Input: part model. Units: mm. Frame: model coordinates. A direction names the side the tool comes from. Coordinates: 2 decimals unless noted, no trailing zeros. Write each loop counter-clockwise with the first axis right and the second up, starting at its lowest first coordinate (ties: lowest second). Pieces come first, ordered by that corner, then holes.
from build123d import *

# Parameters (mm, degrees)
SKETCH1_R           = 3.429
BOSS_EXTRUDE1_DEPTH = 202.2602
BOSS_EXTRUDE2_DEPTH = 6.35
CIRPATTERN1_COUNT   = 2


with BuildPart() as part:
    # Sketch1 → Boss-Extrude1 (new body)
    with BuildSketch(Plane(origin=(0, 0, 0), x_dir=(1, 0, 0), z_dir=(0, 1, 0))):
        with BuildLine():
            Line((19.998392739, 2.54), (-19.998392739, 2.54))
            ThreePointArc((-19.998392739, 2.54), (-31.369, 0), (-19.998392739, -2.54))
            Line((-19.998392739, -2.54), (19.998392739, -2.54))
            ThreePointArc((19.998392739, -2.54), (31.369, 0), (19.998392739, 2.54))
        make_face()
        with Locations(Location((-25.4, 0, 0), (0, 0, 270))):
            Circle(SKETCH1_R, mode=Mode.SUBTRACT)
        with Locations(Location((25.4, 0, 0), (0, 0, 270))):
            Circle(SKETCH1_R, mode=Mode.SUBTRACT)
    extrude(amount=BOSS_EXTRUDE1_DEPTH)

    # Sketch3 → Boss-Extrude2 (add, symmetric)
    with BuildSketch(Plane(origin=(0, 101.1301, 0), x_dir=(1, 0, 0), z_dir=(0, 1, 0))):
        with BuildLine():
            Line((-28.809566389, 4.899369147), (-4.826, 21.59))
            Line((-4.826, 21.59), (4.826, 21.59))
            Line((4.826, 21.59), (28.809566389, 4.899369147))
            ThreePointArc((28.809566389, 4.899369147), (23.85607241, 5.765869284), (19.998392739, 2.54))
            Line((19.998392739, 2.54), (-19.998392739, 2.54))
            ThreePointArc((-19.998392739, 2.54), (-23.85607241, 5.765869284), (-28.809566389, 4.899369147))
        make_face()
    boss_extrude2 = extrude(amount=BOSS_EXTRUDE2_DEPTH, both=True)

    # CirPattern1: Boss-Extrude2 ×2 about axis
    cirpattern1_axis = Axis((0, 0, 0), (0, 1, 0))
    for i in range(1, CIRPATTERN1_COUNT):
        add(boss_extrude2.rotate(cirpattern1_axis, i * 360 / CIRPATTERN1_COUNT))


solid = part.part
Item 1: Pin query (flat end, axial travel): pin 1 Ø8 at (x, y) = (9.5, 24) entering from +Z; pin 2 Ø1 at (x, y) = (-8, 162.5) entering from -Z; pin 3 Ø5.5 at (x, z) = (-14.5, -16.5) entering from +Y. Return the tip coordinate at first contact, or that it passes through.
Item 2: Material intervals for line 1 (X direction, y = 113, z = 0); line 2 (X direction, y = 105.5, z = 0.5); line 3 (X direction, y = 16.5, z = 3), sorted ascending.
Item 3: Access query for faces 1 (the face through (0, 154, 2.54)), 2 (the face through (0, 47, -2.54)), 3 (the face through (0, 107.48, -10)), 4 (the face through (0, 94.78, 10)), 5 (the face through (31.365, 99.714, 0.226)). Directions: +Z, -Z, +X, -X, +Y, -Y. A direction counts if a zero-diameter tool reaches every point of the face in a straight line with its end or side. Return the directions, or none.
Item 4: Section query D-D, the plane x = -1.5. Return loops of the section in (y, z), then the cut area to 3 significant figures.
Item 5: Section query A-A, the plane z = 0. Return loops of the section in (x, y).
Item 6: Section query B-B, the plane y = 132. Return loops of the section in (x, z), then the cut area to 3 significant figures.
Item 7: Pull-direction query (Z, two-part tool) for faces 6 (the face through (22.05, 99.71, -0.74)), 7 (the face through (0, 101, -21.59)), 8 (the face through (0, 94.78, -10)), 9 (the face through (-31.365, 99.714, -0.226)); classes: released by +Z, released by -Z, zero draft, split by the parting line, or undercut.
Item 8: Section query C-C, the plane x = 25.4. Return loops of the section in (y, z).
The answers:
1. pin 1: stops at z = 2.54
1. pin 2: stops at z = -2.54
1. pin 3: stops at y = 107.48
2. line 1: x = -31.37 to -28.83, -21.97 to 21.97, 28.83 to 31.37
2. line 2: x = -31.35 to -28.79, -22.01 to 22.01, 28.79 to 31.35
2. line 3: x = -30.56 to -27.06, -23.74 to -20.24, 20.24 to 23.74, 27.06 to 30.56
3. face 1: +Z, +Y
3. face 2: -Z, -Y
3. face 3: -Z, +Y
3. face 4: +Z, -Y
3. face 5: none
4. outline: (0, -2.54) - (94.78, -2.54) - (94.78, -21.59) - (107.48, -21.59) - (107.48, -2.54) - (202.26, -2.54) - (202.26, 2.54) - (107.48, 2.54) - (107.48, 21.59) - (94.78, 21.59) - (94.78, 2.54) - (0, 2.54) - close
4. area: 1,510 mm2
5. outline: (-31.37, 0) - (-28.83, 0) - (-28.83, 202.26) - (-31.37, 202.26) - close; (-21.97, 0) - (21.97, 0) - (21.97, 202.26) - (-21.97, 202.26) - close; (28.83, 0) - (31.37, 0) - (31.37, 202.26) - (28.83, 202.26) - close
6. outline: (-20, -2.54) - (20, -2.54) arc R5.97 ccw (long way) to (20, 2.54) - (-20, 2.54) arc R5.97 ccw (long way) to start; hole circle Ø6.86 at (-25.4, 0); hole circle Ø6.86 at (25.4, 0)
6. area: 349 mm2
7. face 6: undercut
7. face 7: released by -Z
7. face 8: zero draft
7. face 9: split by the parting line
8. outline: (0, -5.97) - (94.78, -5.97) - (94.78, -7.27) - (107.48, -7.27) - (107.48, -5.97) - (202.26, -5.97) - (202.26, -3.43) - (0, -3.43) - close; (0, 3.43) - (202.26, 3.43) - (202.26, 5.97) - (107.48, 5.97) - (107.48, 7.27) - (94.78, 7.27) - (94.78, 5.97) - (0, 5.97) - close
